from build123d import *

# Parameters (mm, degrees)
F0_R     = 3.5
F1_DEPTH = 12
F2_R     = 2


with BuildPart() as f1:
    # F0 (on Front) → F1 (new body)
    with BuildSketch(Plane.XZ):
        with BuildLine():
            ThreePointArc((-95.075279, 90.171108), (-85.031423, 15.171108), (-95.075279, -59.828892))
            Line((-95.075279, -59.828892), (-5.075279, -59.828892))
            ThreePointArc((-5.075279, -59.828892), (-15.119136, 15.171108), (-5.075279, 90.171108))
            ThreePointArc((-5.075279, 90.171108), (-50.075279, 100.171108), (-95.075279, 90.171108))
        make_face()
        with Locations((-50.075279, 59.171108)):
            Circle(F0_R, mode=Mode.SUBTRACT)
    extrude(amount=F1_DEPTH)

    # F2
    f2_edges = [f1.edges().sort_by_distance(p)[0] for p in [
        (-50.075279, -12, 100.171108),
        (-50.075279, 0, 100.171108),
        (-15.119136, -12, 15.171108),
        (-15.119136, 0, 15.171108),
        (-5.075279, -6, 90.171108),
        (-95.075279, -6, 90.171108),
        (-85.031423, 0, 15.171108),
        (-85.031423, -12, 15.171108),
    ]]
    fillet(f2_edges, radius=F2_R)


solid = f1.part
Geometry check sheet. Reference: the model listing, model coordinates, mm. Coordinates: 2 decimals unless noted, no trailing zeros. One line per item, written item: value.
(1) Release check for a two-part mould opening along Z. For faces 1 (the face through (-49.45, -5.94, 100.17)), 2 (the face through (-51, -6, -59.829)), 3 (the face through (-15.113, -5.944, 13.277)) record: +Z half, -Z half, draft (parallel to the pull), parting line (faces both ways), or undercut.
Data:
face 1: +Z half
face 2: -Z half
face 3: undercut
(2) Depth check by flat-ended pin: pin 1 Ø11 at (x, z) = (-50.08, 59.17) entering from -Y; pin 2 Ø1 at (y, z) = (-11, -28.5) entering from +X; pin 3 Ø4 at (x, y) = (-38.5, -5) entering from +Z; pin 4 Ø5 at (x, y) = (-70, -8) entering from +Z. Enter the tip coordinate at first touch or a pass-through.
Data:
pin 1: stops at y = -12
pin 2: stops at x = -11.8
pin 3: stops at z = 99.74
pin 4: stops at z = 98.73
(3) Thickness scan on probe 1 along X at (y, z) = (-6.75, 60); probe 2 along Z at (x, y) = (-72, -3.5); probe 3 along Z at (x, y) = (-83, -10). Record the ranges inside material, lowest first. Write a range as from..to.
Data:
probe 1: x = -88.58..-53.48, -46.67..-11.57
probe 2: z = -59.83..97.88
probe 3: z = -59.83..94.94
